Read the model definition and answer for the solid it produces. Units are mm, in the model's axes. A direction names the side the tool comes from. Give positions to 0.01 mm unless a question says otherwise; leave off trailing zeros. Write each loop counter-clockwise with the first axis right and the second up, starting at its lowest first coordinate (ties: lowest second). Pieces come first, ordered by that corner, then holes. Notation, with made-up numbers: (61, -11) -> (87, -11) arc R22 ccw to (87, 18) -> close; hole circle Ø6 at (-15, 35.25). An arc over 180 degrees is marked (long way). Use a Markdown table: item, result.
from build123d import *

# Parameters (mm, degrees)
F0_W     = 350
F0_H     = 150
F1_DEPTH = 84
F2_W     = 350
F2_H     = 122
F3_DEPTH = 5
F4_W     = 125
F4_H     = 45
F5_DEPTH = 20
F6_R     = 7.5
F7_DEPTH = 20
F8_R     = 4
F8_R_2   = 1.5
F9_DEPTH = 18
F10_R    = 5
F11_R    = 1


with BuildPart() as f1:
    # F0 (on Top) → F1 (new body)
    with BuildSketch(Plane.XY):
        with Locations((175, 75)):
            Rectangle(F0_W, F0_H)
    extrude(amount=F1_DEPTH)

    # F2 (on face) → F3 (cut)
    with BuildSketch(Plane.XY.offset(84)):
        with Locations((175, 75)):
            Rectangle(F2_W, F2_H)
    extrude(amount=-F3_DEPTH, mode=Mode.SUBTRACT)

    # F4 (on face) → F5 (join)
    with BuildSketch(Plane(origin=(0, 0, 0), x_dir=(0, -1, 0), z_dir=(-1, 0, 0))):
        with Locations((-75, 22.5)):
            Rectangle(F4_W, F4_H)
    extrude(amount=F5_DEPTH)

    # F6 (on face) → F7 (cut)
    with BuildSketch(Plane(origin=(0, 137.5, 0), x_dir=(-1, 0, 0), z_dir=(0, 1, 0))):
        with Locations((10, 31.452831)):
            Circle(F6_R)
    extrude(amount=-F7_DEPTH, mode=Mode.SUBTRACT)

    # F8 (on face) → F9 (join)
    with BuildSketch(Plane(origin=(0, 117.5, 0), x_dir=(-1, 0, 0), z_dir=(0, 1, 0))):
        with Locations((10, 31.452831)):
            Circle(F8_R)
        with Locations((10, 31.452831)):
            Circle(F8_R_2, mode=Mode.SUBTRACT)
    extrude(amount=F9_DEPTH)

    # F10
    f10_edges = [f1.edges().sort_by_distance(p)[0] for p in [
        (175, 150, 84),
        (175, 150, 0),
        (175, 0, 84),
        (175, 0, 0),
        (350, 150, 42),
        (350, 75, 0),
        (350, 75, 79),
        (350, 0, 42),
        (0, 75, 79),
        (0, 150, 42),
        (-20, 75, 45),
        (-20, 75, 0),
    ]]
    fillet(f10_edges, radius=F10_R)

    # F11
    f11_edges = [f1.edges().sort_by_distance(p)[0] for p in [
        (-6, 135.5, 31.452831),
    ]]
    fillet(f11_edges, radius=F11_R)


solid = f1.part
Item 1: Each of these flat-tipped pins is pushed along its axis until it touches: P1, Ø24, axis at x = -10, z = 31.45, coming from the +Y side; P2, Ø2.5, axis at x = -10, z = 31.45, coming from the +Y side; P3, Ø16.5, axis at x = -4, y = 97, coming from the +Z side. Where does it stop, or does it pass through?
Return value:
| item | result |
|---|---|
| P1 | y = 149 |
| P2 | y = 117.5 |
| P3 | z = 78.94 |
Item 2: A tool of negligible diameter and unlimited length cuts with its end or side. For faces 1 (the face through (173, 76, 79)), 2 (the face through (-13, 117.5, 28)), 3 (the face through (-10, 137.5, 17)), 4 (the face through (-10, 12.5, 22)), from which of +Z, -Z, +X, -X, +Y, -Y can it reach the whole face along a straight path? Write none if from no direction.
Return value:
| item | result |
|---|---|
| face 1 | +Z, +X, -X |
| face 2 | +Y |
| face 3 | +Z, -Z, -X, +Y |
| face 4 | +Z, -Z, -X, -Y |
Item 3: For a pull along Y with two mould halves and no side action, classify faces 5 (the face through (-7, 76, 45)), 6 (the face through (173, 14, 81)), 7 (the face through (173, 150, 41)) as +Y half, -Y half, draft (parallel to the pull), parting line (faces both ways), or undercut.
Return value:
| item | result |
|---|---|
| face 5 | draft |
| face 6 | undercut |
| face 7 | +Y half |
Item 4: A cutting plane is placed at B-B (y = 127). Give the vertices of the cut face in (x, z).
Return value:
| item | result |
|---|---|
| outline | (-20, 5) arc R5 ccw to (-15, 0) -> (345, 0) arc R5 ccw to (350, 5) -> (350, 74) arc R5 ccw to (345, 79) -> (5, 79) arc R5 ccw to (0, 74) -> (0, 45) -> (-15, 45) arc R5 ccw to (-20, 40) -> close; circle Ø8 at (-10, 31.45); hole circle Ø15 at (-10, 31.45); hole circle Ø3 at (-10, 31.45) |
Item 5: Straight lines are drawn through the part: line 1 along Z through (x, y) = (-10, 121.75); line 2 along Y through (x, z) = (116.5, 4.5); line 3 along X through (y, z) = (24.5, 53). For each, find the intervals that lie inside material, in ascending order. Write a range as [from, to].
Return value:
| item | result |
|---|---|
| line 1 | [0, 23.95], [27.45, 29.95], [32.95, 35.45], [38.95, 45] |
| line 2 | [0.03, 149.97] |
| line 3 | [0, 350] |
Item 6: A cutting plane is placed at C-C (y = 34.5). Give the vertices of the cut face in (x, z).
Return value:
| item | result |
|---|---|
| outline | (-20, 5) arc R5 ccw to (-15, 0) -> (345, 0) arc R5 ccw to (350, 5) -> (350, 74) arc R5 ccw to (345, 79) -> (5, 79) arc R5 ccw to (0, 74) -> (0, 45) -> (-15, 45) arc R5 ccw to (-20, 40) -> close |
Item 7: A cutting plane is placed at A-A (x = 162.5). Give the vertices of the cut face in (y, z).
Return value:
| item | result |
|---|---|
| outline | (0, 5) arc R5 ccw to (5, 0) -> (145, 0) arc R5 ccw to (150, 5) -> (150, 79) arc R5 ccw to (145, 84) -> (136, 84) -> (136, 79) -> (14, 79) -> (14, 84) -> (5, 84) arc R5 ccw to (0, 79) -> close |
